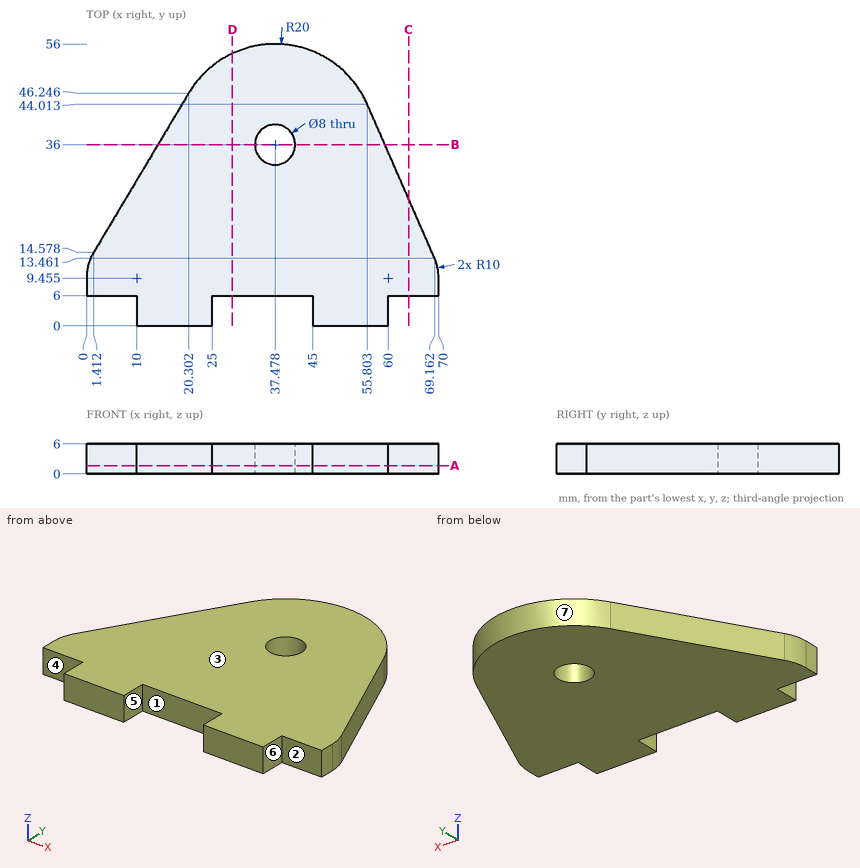
Can you work these out from the drawing? Everything is in mm from the part's minimum corner. A direction names the side the tool comes from. Round coordinates to 2 decimals unless told otherwise and drop trailing zeros. Loops run counter-clockwise (first coordinate to the right, second up) from the corner with the lowest first, then second, coordinate; pieces in that order, holes last. Notation, with made-up numbers: M 50.25,-9 L 61.25,-9 A16 cw 61.25,6 Z; hole C 69.5,56 d2. An arc over 180 degrees is marked long. Answer in a Markdown table with one row per item.
1. If we section it at D-D, the plane x = 29: Please give me the cut outline in (y, z) (1 decimal), plus the area to 3 significant figures.
Established:
| item | result |
|---|---|
| outline | M 6,0 L 54.1,0 L 54.1,6 L 6,6 Z |
| area | 289 mm² |
2. If we section it at C-C, the plane x = 64: Please give me the cut outline in (y, z), plus the area to 3 significant figures.
Established:
| item | result |
|---|---|
| outline | M 6,0 L 25.27,0 L 25.27,6 L 6,6 Z |
| area | 116 mm² |
3. If we section it at A-A, the plane z = 1.65: Please give me the cut outline in (x, y) (1 decimal), plus the area to 3 significant figures.
Established:
| item | result |
|---|---|
| outline | M 0,6 L 10,6 L 10,0 L 25,0 L 25,6 L 45,6 L 45,0 L 60,0 L 60,6 L 70,6 L 70,9.5 A10 ccw 69.2,13.5 L 55.8,44 A20 ccw 20.3,46.2 L 1.4,14.6 A10 ccw 0,9.5 Z; hole C 37.5,36 d8 |
| area | 2,570 mm² |
4. I'm going to push flat-ended pins straight in: pin 1 Ø13 at (x, y) = (37.48, 36) entering from +Z; pin 2 Ø3 at (y, z) = (46, 3) entering from -X; pin 3 Ø1.5 at (y, z) = (18.5, 4.5) entering from +X; pin 4 Ø1.8 at (y, z) = (3, 2.5) entering from +X. Where does each tip first touch, or does it pass through?
Established:
| item | result |
|---|---|
| pin 1 | z = 6 |
| pin 2 | x = 19.26 |
| pin 3 | x = 67.29 |
| pin 4 | x = 60 |
5. On a 3-axis mill with a long thin cutter (end or side, diameter ignored), from which of +Z, -Z, +X, -X, +Y, -Y can I reach the whole of each face in a straight line? I mean the marked faces 1, 2 and 3. Say none if no direction works.
Established:
| item | result |
|---|---|
| face 1 | +Z, -Z, -Y |
| face 2 | +Z, -Z, +X, -Y |
| face 3 | +Z, +X, -X, +Y, -Y |
6. If we section it at B-B, the plane y = 36: Please give me the cut outline in (x, z).
Established:
| item | result |
|---|---|
| outline | M 14.19,0 L 33.48,0 L 33.48,6 L 14.19,6 Z; M 41.48,0 L 59.31,0 L 59.31,6 L 41.48,6 Z |
7. Thinking about a two-plate mould opening in X: for the marked faces 4, 5, 6 and 7, which applies, pulls with the +X half, pulls with the -X half, needs draft (parallel to the pull), parting line crosses it, or undercut?
Established:
| item | result |
|---|---|
| face 4 | needs draft |
| face 5 | undercut |
| face 6 | pulls with the +X half |
| face 7 | parting line crosses it |
8. Please list where these lines run through material, in increasing order: line 1 (X direction, y = 10, z = 4.45) (1 decimal); line 2 (Y direction, x = 40.5, z = 1.3); line 3 (Y direction, x = 8, z = 1.55) (1 decimal). Write a range as from..to.
Established:
| item | result |
|---|---|
| line 1 | 0..70 |
| line 2 | 6..33.38, 38.62..55.77 |
| line 3 | 6..25.6 |
